Answer from the drawing. Dimensions are ordinates in mm from the lowest x, y and z of the part. Coordinates: 2 decimals unless noted, no trailing zeros. Order: outer loops, then holes, each group sorted by start corner. A loop starts at its lowest first (then second) coordinate and runs counter-clockwise, first axis right, second up.
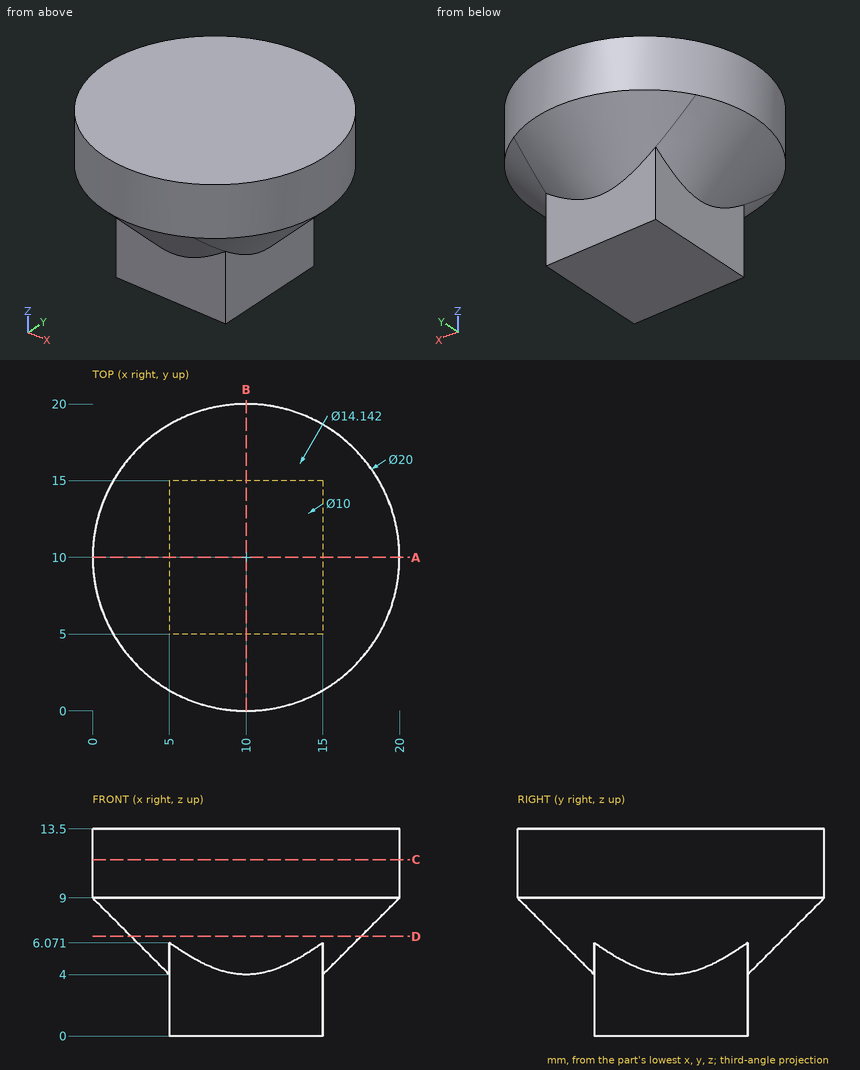
1) Section A-A (y = 10) is taken. Give the vertices of the cut face in (x, z), then the cut area to 3 significant figures.
2) Section C-C (z = 11.5) is taken. Give the vertices of the cut face in (x, y), then the cut area to 3 significant figures.
3) Each of these flat-tipped pins is pushed along its axis until it touches: P1, Ø3, axis at x = 13, z = 10, coming from the +Y side; P2, Ø5, axis at y = 10, z = 2, coming from the +X side; P3, Ø5, axis at y = 12, z = 3, coming from the -X side. Where does it stop, or does it pass through?
4) Section D-D (z = 6.5) is taken. Give the vertices of the cut face in (x, y).
5) Consider L1, parallel to Y at x = 12.5, z = 2; L2, parallel to X at y = 9, z = 7.25. Determine where each line is inside the solid, lowest interval first.
Filled sheet:
1. outline: (0, 9) - (5, 4) - (5, 0) - (15, 0) - (15, 4) - (20, 9) - (20, 13.5) - (0, 13.5) - close
1. area: 205 mm2
2. outline: circle Ø20 at (10, 10)
2. area: 314 mm2
3. P1: stops at y = 19.89
3. P2: stops at x = 15.5
3. P3: stops at x = 3.73
4. outline: circle Ø15 at (10, 10)
5. L1: y = 5 to 15
5. L2: x = 1.81 to 18.19
